Read the model definition and answer for the solid it produces. Units are mm, in the model's axes. A direction names the side the tool comes from. Coordinates: 2 decimals unless noted, no trailing zeros. Loops run counter-clockwise (first coordinate to the right, second up) from the corner with the lowest first, then second, coordinate; pieces in that order, holes last. Notation, with made-up numbers: (30, 30.5) -> (44, 30.5) arc R27 ccw to (44, 59.5) -> close; hole circle Ø2 at (38, 23). An arc over 180 degrees is marked (long way). Answer as a JSON object with one key per item and string values. Group by question number.
Q1. Each of these flat-tipped pins is pushed along its axis until it touches: P1, Ø3, axis at x = -2, y = -0.5, coming from the -Z side; P2, Ø1.5, axis at x = 4.5, z = 2.5, coming from the -Y side; P3, Ø0.6, axis at x = 0, y = -2, coming from the -Z side. Where does it stop, or does it pass through?
Q2. The part is cut by section B-B on x = 2.25. Write down the section's boundary in (y, z).
Q3. The part is cut by section A-A on y = 0.25. Write down the section's boundary in (x, z), and give its area (3 significant figures).
Q4. For faces 5 (the flat face through (0, -2, 1)), 6 (the flat face through (5, 1, 1.5)), 7 (the flat face through (-5, 1, 1.5)), determine the directions among +Z, -Z, +X, -X, +Y, -Y from which every point of the face is accessible in a straight line to the end or side of a thin tool.
Q5. Determine the mould class of faces 1 (the flat face through (-0.1, -1.25, 0.7)), 2 (the cylindrical face through (3.999, 1.031, 2.715)), 3 (the flat face through (0, 1, 0.5)), 4 (the flat face through (-5.8, 1, 1)) for opening direction X: released by +X, released by -X, zero draft, split by the parting line, or undercut.
Q6. Straight lines are drawn through the part: line 1 along Z through (x, y) = (4.5, -0.25); line 2 along Y through (x, z) = (3.75, 0.6); line 3 along X through (y, z) = (0.75, 1.8). For each, find the intervals that lie inside material, in ascending order. Write a range as [from, to].
Q7. The part is cut by section C-C on x = -4.5. Write down the section's boundary in (y, z), and give its area (3 significant figures).
from build123d import *

# Parameters (mm, degrees)
SKETCH_1_W          = 8.6
SKETCH_1_H          = 6.5
EXTRUDE_1_DEPTH     = 3
FILLET_1_R          = 2
SKETCH_2_W          = 1.5
SKETCH_2_H          = 4.5
EXTRUDE_2_DEPTH     = 1.5
SKETCH_3_W          = 1.5
SKETCH_3_H          = 4.5
EXTRUDE_3_DEPTH     = 1.5
FILLET_2_R          = 1
FILLET_3_R          = 1
CUT_EXTRUDE_1_DEPTH = 1
SKETCH_5_W          = 10
SKETCH_5_H          = 4.5
CUT_EXTRUDE_2_DEPTH = 0.5


with BuildPart() as part:
    # 草图1 → 凸台-拉伸1 (new body)
    with BuildSketch(Plane.XY):
        Rectangle(SKETCH_1_W, SKETCH_1_H)
    extrude(amount=EXTRUDE_1_DEPTH)

    # 圆角1
    fillet_1_edges = [part.edges().sort_by_distance(p)[0] for p in [
        (0, -3.25, 3),
    ]]
    fillet(fillet_1_edges, radius=FILLET_1_R)

    # 草图2 → 凸台-拉伸2 (add)
    with BuildSketch(Plane(origin=(4.3, 0, 0), x_dir=(0, 0, -1), z_dir=(1, 0, 0))):
        with Locations((-0.75, 1)):
            Rectangle(SKETCH_2_W, SKETCH_2_H)
    extrude(amount=EXTRUDE_2_DEPTH)

    # 草图3 → 凸台-拉伸3 (add)
    with BuildSketch(Plane.ZY.offset(4.3)):
        with Locations((0.75, 1)):
            Rectangle(SKETCH_3_W, SKETCH_3_H)
    extrude(amount=EXTRUDE_3_DEPTH)

    # 圆角2
    fillet_2_edges = [part.edges().sort_by_distance(p)[0] for p in [
        (4.3, 1, 3),
        (4.3, -3.25, 0.5),
        (4.3, -2.664213562, 2.414213562),
    ]]
    fillet(fillet_2_edges, radius=FILLET_2_R)

    # 圆角3
    fillet_3_edges = [part.edges().sort_by_distance(p)[0] for p in [
        (-4.3, 1, 3),
        (-4.3, -3.25, 0.5),
        (-4.3, -2.664213562, 2.414213562),
    ]]
    fillet(fillet_3_edges, radius=FILLET_3_R)

    # 草图4 → 切除-拉伸1 (cut)
    with BuildSketch(Plane(origin=(0, 0, 0), x_dir=(-1, 0, 0), z_dir=(0, 0, -1))):
        with BuildLine():
            Line((-4.3, -1.25), (-4.3, -2.25))
            ThreePointArc((-4.3, -2.25), (-4.007106781, -2.957106781), (-3.3, -3.25))
            Line((-3.3, -3.25), (3.3, -3.25))
            ThreePointArc((3.3, -3.25), (4.007106781, -2.957106781), (4.3, -2.25))
            Line((4.3, -2.25), (4.3, -1.25))
            Line((4.3, -1.25), (-4.3, -1.25))
        make_face()
    extrude(amount=-CUT_EXTRUDE_1_DEPTH, mode=Mode.SUBTRACT)

    # 草图5 → 切除-拉伸2 (cut)
    with BuildSketch(Plane(origin=(0, 0, 0), x_dir=(-1, 0, 0), z_dir=(0, 0, -1))):
        with Locations((0, 1)):
            Rectangle(SKETCH_5_W, SKETCH_5_H)
    extrude(amount=-CUT_EXTRUDE_2_DEPTH, mode=Mode.SUBTRACT)


solid = part.part
Final values:
{
 "1": {"P1": "stops at z = 0.5", "P2": "stops at y = -2.71", "P3": "stops at z = 1"},
 "2": {"outline": "(-3.25, 1) -> (-1.25, 1) -> (-1.25, 0.5) -> (3.25, 0.5) -> (3.25, 3) -> (-1.25, 3) arc R2 ccw to start"},
 "3": {"outline": "(-5.8, 0) -> (-5, 0) -> (-5, 0.5) -> (5, 0.5) -> (5, 0) -> (5.8, 0) -> (5.8, 1.5) -> (4.3, 1.5) -> (4.3, 2) arc R1 ccw to (3.3, 3) -> (-3.3, 3) arc R1 ccw to (-4.3, 2) -> (-4.3, 1.5) -> (-5.8, 1.5) -> close", "area": "24.9 mm2"},
 "4": {"face 5": "-Z, +X, -X, -Y", "face 6": "+Z, +X, +Y, -Y", "face 7": "+Z, -X, +Y, -Y"},
 "5": {"face 1": "zero draft", "face 2": "released by +X", "face 3": "undercut", "face 4": "released by -X"},
 "6": {"line 1": "z = [0.5, 1.5]", "line 2": "y = [-1.25, 3.25]", "line 3": "x = [-4.3, 4.3]"},
 "7": {"outline": "(-1.25, 0.5) -> (3.25, 0.5) -> (3.25, 1.5) -> (-1.25, 1.5) -> close", "area": "4.50 mm2"}
}
